```python
from build123d import *

# Parameters (mm, degrees)
SKETCH_1_W          = 20
SKETCH_1_H          = 20
EXTRUDE_1_DEPTH     = 120
SKETCH_2_W          = 10
SKETCH_2_H          = 20
CUT_EXTRUDE_1_DEPTH = 120
CUT_EXTRUDE_2_DEPTH = 120
SKETCH_4_R          = 3
CUT_EXTRUDE_3_DEPTH = 2
SKETCH_8_W          = 19.6
SKETCH_8_H          = 0.2
SKETCH_8_W_2        = 0.2
SKETCH_8_H_2        = 19.6
CUT_EXTRUDE_6_DEPTH = 15
SKETCH_9_W          = 10
SKETCH_9_H          = 20
CUT_EXTRUDE_7_DEPTH = 20
SKETCH_10_W         = 19.6
SKETCH_10_H         = 19.6
EXTRUDE_2_DEPTH     = 15
CUT_EXTRUDE_8_DEPTH = 20
CUT_EXTRUDE_9_DEPTH = 20


with BuildPart() as part:
    # 草图1 → 凸台-拉伸1 (new body)
    with BuildSketch(Plane.XY):
        with Locations((10, 10)):
            Rectangle(SKETCH_1_W, SKETCH_1_H)
    extrude(amount=EXTRUDE_1_DEPTH)

    # 草图2 → 切除-拉伸1 (cut)
    with BuildSketch(Plane(origin=(0, 20, 0), x_dir=(1, 0, 0), z_dir=(0, 1, 0))):
        with Locations((15, -10)):
            Rectangle(SKETCH_2_W, SKETCH_2_H)
    extrude(amount=-CUT_EXTRUDE_1_DEPTH, mode=Mode.SUBTRACT)

    # 草图3 → 切除-拉伸2 (cut)
    with BuildSketch(Plane(origin=(10, 0, 0), x_dir=(0, 0, -1), z_dir=(1, 0, 0))):
        with BuildLine():
            ThreePointArc((-8.45, 10), (-9.40684068, 11.432013275), (-11.096015511, 11.096015511))
            Line((-11.096015511, 11.096015511), (-8.903984489, 8.903984489))
            ThreePointArc((-8.903984489, 8.903984489), (-8.567986725, 9.40684068), (-8.45, 10))
        make_face()
        with BuildLine():
            Line((-8.903984489, 8.903984489), (-11.096015511, 11.096015511))
            ThreePointArc((-11.096015511, 11.096015511), (-11.096015511, 8.903984489), (-8.903984489, 8.903984489))
        make_face()
    extrude(amount=-CUT_EXTRUDE_2_DEPTH, mode=Mode.SUBTRACT)

    # 草图4 → 切除-拉伸3 (cut)
    with BuildSketch(Plane.ZY):
        with Locations((10, 10)):
            Circle(SKETCH_4_R)
    extrude(amount=-CUT_EXTRUDE_3_DEPTH, mode=Mode.SUBTRACT)

    # 草图8 → 切除-拉伸6 (cut)
    with BuildSketch(Plane.XY.offset(120)):
        with Locations((10, 19.9)):
            Rectangle(SKETCH_8_W, SKETCH_8_H)
        with Locations((0.1, 19.9)):
            Rectangle(SKETCH_8_W_2, SKETCH_8_H)
        with Locations((0.1, 10)):
            Rectangle(SKETCH_8_W_2, SKETCH_8_H_2)
        with Locations((19.9, 10)):
            Rectangle(SKETCH_8_W_2, SKETCH_8_H_2)
        with Locations((19.9, 0.1)):
            Rectangle(SKETCH_8_W_2, SKETCH_8_H)
        with Locations((10, 0.1)):
            Rectangle(SKETCH_8_W, SKETCH_8_H)
        with Locations((0.1, 0.1)):
            Rectangle(SKETCH_8_W_2, SKETCH_8_H)
        with Locations((19.9, 19.9)):
            Rectangle(SKETCH_8_W_2, SKETCH_8_H)
    extrude(amount=-CUT_EXTRUDE_6_DEPTH, mode=Mode.SUBTRACT)

    # 草图9 → 切除-拉伸7 (cut)
    with BuildSketch(Plane(origin=(0, 20, 0), x_dir=(1, 0, 0), z_dir=(0, 1, 0))):
        Polygon((0, 0), (0, -45), (20, -45), (20, -20), (10, -20), (10, 0), align=None)
        with Locations((15, -10)):
            Rectangle(SKETCH_9_W, SKETCH_9_H)
    extrude(amount=-CUT_EXTRUDE_7_DEPTH, mode=Mode.SUBTRACT)

    # 草图10 → 凸台-拉伸2 (add)
    with BuildSketch(Plane(origin=(0, 0, 45), x_dir=(-1, 0, 0), z_dir=(0, 0, -1))):
        with Locations((-10, 10)):
            Rectangle(SKETCH_10_W, SKETCH_10_H)
    extrude(amount=EXTRUDE_2_DEPTH)

    # 草图11 → 切除-拉伸8 (cut)
    with BuildSketch(Plane(origin=(0, 19.8, 0), x_dir=(1, 0, 0), z_dir=(0, 1, 0))):
        with BuildLine():
            ThreePointArc((11.547573501, -112.5), (10.487812185, -111.029569439), (8.757681845, -111.569855559))
            Line((8.757681845, -111.569855559), (11.237465157, -113.430144441))
            ThreePointArc((11.237465157, -113.430144441), (11.468004062, -112.990238683), (11.547573501, -112.5))
        make_face()
        with BuildLine():
            Line((11.237465157, -113.430144441), (8.757681845, -111.569855559))
            ThreePointArc((8.757681845, -111.569855559), (9.06742906, -113.739891656), (11.237465157, -113.430144441))
        make_face()
    extrude(amount=-CUT_EXTRUDE_8_DEPTH, mode=Mode.SUBTRACT)

    # 草图12 → 切除-拉伸9 (cut)
    with BuildSketch(Plane(origin=(0, 19.8, 0), x_dir=(1, 0, 0), z_dir=(0, 1, 0))):
        with BuildLine():
            ThreePointArc((11.55, -37.5), (10.490153037, -36.029540888), (8.76, -36.57))
            Line((8.76, -36.57), (11.24, -38.43))
            ThreePointArc((11.24, -38.43), (11.470459112, -37.990153037), (11.55, -37.5))
        make_face()
        with BuildLine():
            Line((11.24, -38.43), (8.76, -36.57))
            ThreePointArc((8.76, -36.57), (9.07, -38.74), (11.24, -38.43))
        make_face()
    extrude(amount=-CUT_EXTRUDE_9_DEPTH, mode=Mode.SUBTRACT)


solid = part.part
```
CAD build for the part. Positions are in the model's coordinates, mm. A direction names the side the tool comes from. Round coordinates to 2 decimals unless told otherwise and drop trailing zeros. Loops run counter-clockwise (first coordinate to the right, second up) from the corner with the lowest first, then second, coordinate; pieces in that order, holes last. Notation, with made-up numbers: (64.5, -19) - (96.5, -19) arc R22 cw to (96.5, 17) - close; hole circle Ø4 at (23, -9.75). An arc over 180 degrees is marked (long way). Return JSON: item names as keys, results as strings. Group by question number.
Q1. Band-saw the part on A-A on x = 10. Give the cut face in (y, z), plus the area to 3 significant figures.
Q2. Drill centre lines: line 1 along Z through (x, y) = (11.25, 12.75); line 2 along Z through (x, y) = (10, 12.5); line 3 along X through (y, z) = (17.5, 35.5). Where is each one in solid material? Low to high. Write a range as [from, to].
Q3. Flat gauge pins, fed straight in: pin 1 Ø4.5 at (x, z) = (12, 115) entering from -Y; pin 2 Ø12 at (x, z) = (9.5, 35) entering from +Y; pin 3 Ø12 at (y, z) = (12, 38) entering from +X. Where does each tip first touch, or does it go through?
Q4. Band-saw the part on B-B on y = 11. Give the cut face in (x, z).
Q5. Tool access for faces 1 (the face through (19.8, 10, 38)), 2 (the face through (9.9, 19.8, 114.3)), 3 (the face through (10.1, 19.8, 39.3)), 4 (the face through (0.2, 10, 38)), 5 (the face through (10.1, 0.2, 39.3)): list every direction of +Z, -Z, +X, -X, +Y, -Y with a clear straight run to the whole face (end or side of a thin tool).
Q6. Band-saw the part on C-C on z = 40. Give the cut face in (x, y).
Solutions:
{
 "1": {"outline": "(0, 45) - (0.2, 45) - (0.2, 39.05) - (19.8, 39.05) - (19.8, 45) - (20, 45) - (20, 105) - (19.8, 105) - (19.8, 110.95) - (0.2, 110.95) - (0.2, 105) - (0, 105) - close; (0.2, 30) - (19.8, 30) - (19.8, 35.95) - (0.2, 35.95) - close; (0.2, 114.05) - (19.8, 114.05) - (19.8, 120) - (0.2, 120) - close", "area": "1,670 mm^2"},
 "2": {"line 1": "z = [30, 36.58], [38.42, 111.59], [113.41, 120]", "line 2": "z = [30, 35.95], [39.05, 110.95], [114.05, 120]", "line 3": "x = [0.2, 19.8]"},
 "3": {"pin 1": "stops at y = 0.2", "pin 2": "stops at y = 19.8", "pin 3": "stops at x = 19.8"},
 "4": {"outline": "(0, 45) - (0.2, 45) - (0.2, 30) - (19.8, 30) - (19.8, 45) - (20, 45) - (20, 105) - (19.8, 105) - (19.8, 120) - (0.2, 120) - (0.2, 105) - (0, 105) - close; hole circle Ø3.1 at (10, 37.5); hole circle Ø3.1 at (10, 112.5)"},
 "5": {"face 1": "-Z, +X, +Y, -Y", "face 2": "+Z, +X, -X, +Y", "face 3": "-Z, +X, -X, +Y", "face 4": "-Z, -X, +Y, -Y", "face 5": "-Z, +X, -X, -Y"},
 "6": {"outline": "(0.2, 0.2) - (19.8, 0.2) - (19.8, 19.8) - (0.2, 19.8) - close"}
}
